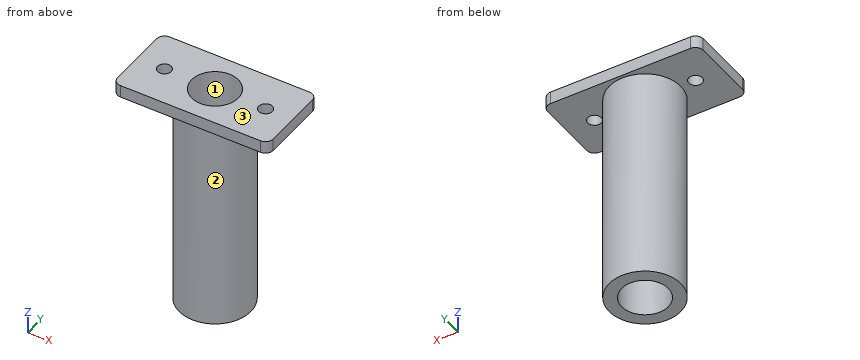
Autodesk Fusion 360 part; units mm, degrees
sketch "support" plane through (0, 0, 0) normal (0, 0, 1) x (1, 0, 0)
  line L0 (20, 10) -> (-20, 10)
  line L1 (-20, 10) -> (-20, -10)
  line L2 (-20, -10) -> (20, -10)
  line L3 (20, -10) -> (20, 10)
  line L4 (20, 10) -> (-20, -10) construction
  line L5 (-20, 10) -> (20, -10) construction
  circle A0 centre (0, 0) radius 6
  line L6 (-20, 0) -> (20, 0)
  circle A1 centre (-13, 0) radius 1.75
  line L7 (0, 10) -> (0, -10)
  circle A2 centre (13, 0) radius 1.75
  circle A3 centre (0, 0) radius 9.2
  dimension "d1" = 40
  dimension "d2" = 20
  dimension "d3" = 12
  dimension "d4" = 3.5
  dimension "d5" = 7
  dimension "d10" = 3.2
extrude "Extrude1" add sketch "support" along normal blind 3.2 contours L0 L3 L6 L7 A2 A3 | L0 L1 L6 A1 L7 A3 | L2 L3 L6 L7 A2 A3 | A0 L6 L7 A3 | A0 L6 L7 A3 | L1 L2 L6 A1 L7 A3 | A0 L6 L7 A3 | A0 L6 L7 A3
extrude "Extrude3" add sketch "support" against normal blind 55 contours A0 L6 L7 A3 | A0 L6 L7 A3 | A0 L6 L7 A3 | A0 L6 L7 A3
fillet "Fillet1" radius 2 4 edges at (20, 10, 1.6) (20, -10, 1.6) (-20, 10, 1.6) (-20, -10, 1.6)
Source: CAD feature listing. Evaluate the final solid. Frame: model axes, mm. Face numbers are marked on the shaded views. Give positions to 0.01 mm unless a question says otherwise; leave off trailing zeros. Order: outer loops, then holes, each group sorted by start corner. A loop starts at its lowest first (then second) coordinate and runs counter-clockwise, first axis right, second up. Notation, with made-up numbers: (-10, -19.75) -> (-4, -19.75) arc R13 ccw to (-4, -0.75) -> close; hole circle Ø5 at (64.25, -25.75). An arc over 180 degrees is marked (long way). Use a Markdown table: item, result.
Q1. Section A-A (y = 0). Return the cut outline in (x, z), and give its area (3 significant figures).
A:
| item | result |
|---|---|
| outline | (-20, 0) -> (-14.75, 0) -> (-14.75, 3.2) -> (-20, 3.2) -> close; (-11.25, 0) -> (-9.2, 0) -> (-9.2, -55) -> (-6, -55) -> (-6, 3.2) -> (-11.25, 3.2) -> close; (6, -55) -> (9.2, -55) -> (9.2, 0) -> (11.25, 0) -> (11.25, 3.2) -> (6, 3.2) -> close; (14.75, 0) -> (20, 0) -> (20, 3.2) -> (14.75, 3.2) -> close |
| area | 419 mm^2 |
Q2. Material intervals for line 1 (X direction, y = 0, z = 1.45); line 2 (X direction, y = 0, z = -28.5); line 3 (Y direction, x = -13, z = 1.55), sorted ascending. Write a range as [from, to].
A:
| item | result |
|---|---|
| line 1 | [-20, -14.75], [-11.25, -6], [6, 11.25], [14.75, 20] |
| line 2 | [-9.2, -6], [6, 9.2] |
| line 3 | [-10, -1.75], [1.75, 10] |
Q3. Pull-direction query (Y, two-part tool) for the marked faces 1, 2 and 3; classes: +Y half, -Y half, draft (parallel to the pull), parting line (faces both ways), or undercut.
A:
| item | result |
|---|---|
| face 1 | undercut |
| face 2 | parting line |
| face 3 | draft |
Q4. Section C-C (y = 2.75). Return the cut outline in (x, z).
A:
| item | result |
|---|---|
| outline | (-20, 0) -> (-8.78, 0) -> (-8.78, -55) -> (-5.33, -55) -> (-5.33, 3.2) -> (-20, 3.2) -> close; (5.33, -55) -> (8.78, -55) -> (8.78, 0) -> (20, 0) -> (20, 3.2) -> (5.33, 3.2) -> close |
Q5. First-contact query: P1, Ø5, axis at x = 4.5, z = -22, coming from the +Y side; P2, Ø9.5, axis at x = 0, y = 0, coming from the +Z side; P3, Ø10, axis at y = 7.5, z = -7, coming from the -X side; P4, Ø3, axis at x = 1, z = -38, coming from the +Y side. Flat tips, straight axial feed; report the tip coordinate or a pass-through.
A:
| item | result |
|---|---|
| P1 | y = 8.98 |
| P2 | through |
| P3 | x = -8.85 |
| P4 | y = 9.2 |
Q6. Section D-D (z = -14.5). Return the cut outline in (x, y).
A:
| item | result |
|---|---|
| outline | circle Ø18.4 at (0, 0); hole circle Ø12 at (0, 0) |
Q7. Section B-B (x = -13). Return the cut outline in (y, z).
A:
| item | result |
|---|---|
| outline | (-10, 0) -> (-1.75, 0) -> (-1.75, 3.2) -> (-10, 3.2) -> close; (1.75, 0) -> (10, 0) -> (10, 3.2) -> (1.75, 3.2) -> close |
